from build123d import *

# Parameters (mm, degrees)
F1_W     = 65
F1_H     = 40
F1_W_2   = 8
F1_H_2   = 3
F1_R     = 1.5
F1_W_3   = 16
F1_H_3   = 3.5
F2_DEPTH = 3
F4_D     = 2.4
F5_W     = 12
F5_H     = 7.5
F6_DEPTH = 25
F7_R     = 5


with BuildPart() as f2:
    # F1 (on Top) → F2 (new body)
    with BuildSketch(Plane.XY):
        Rectangle(F1_W, F1_H)
        with Locations((-24, -14)):
            Rectangle(F1_W_2, F1_H_2, mode=Mode.SUBTRACT)
        with Locations((-14.5, -14)):
            Circle(F1_R, mode=Mode.SUBTRACT)
        with Locations((0, -10.75)):
            Rectangle(F1_W_3, F1_H_3, mode=Mode.SUBTRACT)
        with Locations((14.5, -14)):
            Circle(F1_R, mode=Mode.SUBTRACT)
        with Locations((24, -14)):
            Rectangle(F1_W_2, F1_H_2, mode=Mode.SUBTRACT)
        with Locations((-24, 14)):
            Rectangle(F1_W_2, F1_H_2, mode=Mode.SUBTRACT)
        with Locations((-14.5, 14)):
            Circle(F1_R, mode=Mode.SUBTRACT)
        with Locations((14.5, 14)):
            Circle(F1_R, mode=Mode.SUBTRACT)
        with Locations((24, 14)):
            Rectangle(F1_W_2, F1_H_2, mode=Mode.SUBTRACT)
    extrude(amount=F2_DEPTH)

    # F4 (through all)
    with Locations(Plane.XY.offset(3)):
        with Locations((-30, 4), (-30, -4), (-18, 4), (-18, -4), (18, 4), (18, -4), (30, 4), (30, -4)):
            Hole(F4_D / 2)

    # F5 (on face) → F6 (cut)
    with BuildSketch(Plane.XY.offset(3)):
        with Locations((0, 16.25)):
            Rectangle(F5_W, F5_H)
    extrude(amount=-F6_DEPTH, mode=Mode.SUBTRACT)

    # F7
    f7_edges = [f2.edges().sort_by_distance(p)[0] for p in [
        (-32.5, -20, 1.5),
        (-32.5, 20, 1.5),
        (32.5, -20, 1.5),
        (32.5, 20, 1.5),
        (-6, 20, 1.5),
        (6, 20, 1.5),
    ]]
    fillet(f7_edges, radius=F7_R)


solid = f2.part
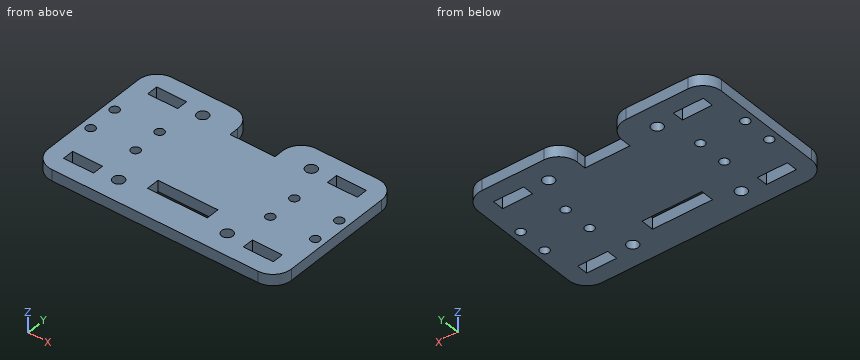
Design review of the part built by this model. Coordinates are the model's own, in mm. Round coordinates to 2 decimals unless told otherwise and drop trailing zeros. Loops run counter-clockwise (first coordinate to the right, second up) from the corner with the lowest first, then second, coordinate; pieces in that order, holes last. Notation, with made-up numbers: M 58.5,53 L 114.5,53 A29 ccw 114.5,88 Z; hole C 51.25,59 d5. An arc over 180 degrees is marked long. Answer as a JSON object with one key per item and string values.
Item 1: We need section C-C on x = 3.5. Give the boundary of the cut face in (y, z).
Answer sheet:
{"outline": "M -20,0 L -12.5,0 L -12.5,3 L -20,3 Z; M -9,0 L 12.5,0 L 12.5,3 L -9,3 Z"}
Item 2: We need section B-B on x = -18. Give the boundary of the cut face in (y, z).
Answer sheet:
{"outline": "M -20,0 L -5.2,0 L -5.2,3 L -20,3 Z; M -2.8,0 L 2.8,0 L 2.8,3 L -2.8,3 Z; M 5.2,0 L 20,0 L 20,3 L 5.2,3 Z"}
Item 3: We need section D-D on y = -4. Give the boundary of the cut face in (x, z), and give its area (3 significant figures).
Answer sheet:
{"outline": "M -32.5,0 L -31.2,0 L -31.2,3 L -32.5,3 Z; M -28.8,0 L -19.2,0 L -19.2,3 L -28.8,3 Z; M -16.8,0 L 16.8,0 L 16.8,3 L -16.8,3 Z; M 19.2,0 L 28.8,0 L 28.8,3 L 19.2,3 Z; M 31.2,0 L 32.5,0 L 32.5,3 L 31.2,3 Z", "area": "166 mm^2"}
Item 4: We need section A-A on y = 14. Give the boundary of the cut face in (x, z), and give its area (3 significant figures).
Answer sheet:
{"outline": "M -32.5,0 L -28,0 L -28,3 L -32.5,3 Z; M -20,0 L -16,0 L -16,3 L -20,3 Z; M -13,0 L -6,0 L -6,3 L -13,3 Z; M 6,0 L 13,0 L 13,3 L 6,3 Z; M 16,0 L 20,0 L 20,3 L 16,3 Z; M 28,0 L 32.5,0 L 32.5,3 L 28,3 Z", "area": "93.0 mm^2"}
Item 5: Wall thickness on L1, parallel to Y at x = -14.5, z = 1.65; L2, parallel to X at y = -9.5, z = 2.1; L3, parallel to X at y = 3, z = 2.55: over which ranges is each line inside the solid? List them lowest first. Write a range as from..to.
Answer sheet:
{"L1": "y = -20..-15.5, -12.5..12.5, 15.5..20", "L2": "x = -32.5..-8, 8..32.5", "L3": "x = -32.5..-30.66, -29.34..-18.66, -17.34..17.34, 18.66..29.34, 30.66..32.5"}
Item 6: Clearance check with a flat-ended pin moving along its axis: P1, Ø1.4, axis at x = -30, y = 4, coming from the +Z side. State where the tip first meets the part, or that it passes through.
Answer sheet:
{"P1": "passes through"}
